Could you check a few things on this drawing? It's one solid part, dimensions in mm from its lowest x, y, z. Coordinates: 2 decimals unless noted, no trailing zeros. Loops run counter-clockwise (first coordinate to the right, second up) from the corner with the lowest first, then second, coordinate; pieces in that order, holes last.
1) Will these pins go through, and if not, where does the flat tip stop? P1, Ø1, axis at x = 1.5, y = 1.5, coming from the -Z side; P2, Ø1.5, axis at x = 5.5, z = 2.5, coming from the +Y side.
2) Imagine slicing it at B-B on x = 5.25. Please give me the cut outline in (y, z) (1 decimal).
3) Imagine slicing it at A-A on z = 3.05. Give the number of separate pieces and of enclosed holes in the cut face, plus the area to 3 significant figures.
4) If I drill on line 1 along X through (y, z) = (2.8, 1.1) (1 decimal); line 2 along Y through (x, z) = (10, 0.65) (1 decimal); line 3 along Z through (x, y) = (8.5, 1.5), over which ranges is the centre line in solid material (lowest first)?
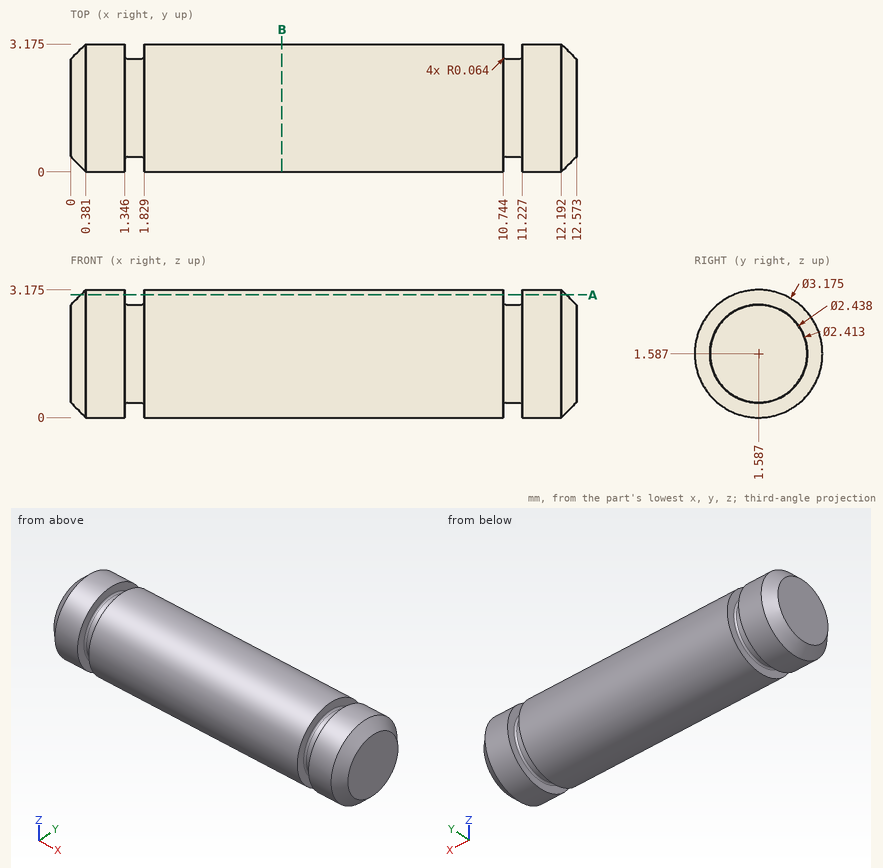
Filled in:
1. P1: stops at z = 0
1. P2: stops at y = 3.17
2. outline: circle Ø3.2 at (1.6, 1.6)
3. separate pieces: 3
3. enclosed holes: 0
3. area: 13.6 mm2
4. line 1: x = 0.1 to 1.3, 1.8 to 10.7, 11.2 to 12.5
4. line 2: y = 0.3 to 2.9
4. line 3: z = 0 to 3.17
